Input: part model. Units: mm. Frame: model coordinates. Face numbers are marked on the shaded views. A direction names the side the tool comes from. Round coordinates to 2 decimals unless told otherwise and drop trailing zeros. Order: outer loops, then holes, each group sorted by start corner. A loop starts at its lowest first (then second) coordinate and runs counter-clockwise, first axis right, second up. Notation, with made-up numbers: (87, 27.5) - (129, 27.5) arc R18 cw to (129, 39.5) - close; hole circle Ø7 at (-3, -24.5). An arc over 180 degrees is marked (long way). One line per item, written item: value. Start each with the question number.
from build123d import *

# Parameters (mm, degrees)
F0_R      = 37.5
F0_R_2    = 23.25
F1_DEPTH  = 2.6
F2_R      = 28.25
F2_R_2    = 23.25
F3_DEPTH  = 10
F4_SIZE   = 2
F5_R      = 23.25
F5_R_2    = 4.25
F6_DEPTH  = 2.6
F8_DEPTH  = 2.601
F10_DEPTH = 2.601


with BuildPart() as f1:
    # F0 (on Top) → F1 (new body)
    with BuildSketch(Plane.XY):
        Circle(F0_R)
        Circle(F0_R_2, mode=Mode.SUBTRACT)
    extrude(amount=F1_DEPTH)

    # F2 (on face) → F3 (join)
    with BuildSketch(Plane.XY.offset(2.6)):
        Circle(F2_R)
        Circle(F2_R_2, mode=Mode.SUBTRACT)
    extrude(amount=F3_DEPTH)

    # F4
    f4_edges = [f1.edges().sort_by_distance(p)[0] for p in [
        (-28.25, 0, 12.6),
    ]]
    chamfer(f4_edges, length=F4_SIZE)

    # F5 (on Top) → F6 (join)
    with BuildSketch(Plane.XY):
        Circle(F5_R)
        Circle(F5_R_2, mode=Mode.SUBTRACT)
    extrude(amount=F6_DEPTH)

    # F7 (on face) → F8 (cut, through all)
    with BuildSketch(Plane.XY.offset(2.6)):
        with BuildLine():
            ThreePointArc((-3.877788, 8.121746), (0, 9), (3.877788, 8.121746))
            ThreePointArc((3.877788, 8.121746), (5.806341, 7.897177), (7.468517, 8.900632))
            Line((7.468517, 8.900632), (10.1022, 12.039333))
            ThreePointArc((10.1022, 12.039333), (10.754749, 14.509432), (9.267329, 16.586639))
            ThreePointArc((9.267329, 16.586639), (0, 19), (-9.267329, 16.586639))
            ThreePointArc((-9.267329, 16.586639), (-10.754749, 14.509432), (-10.1022, 12.039333))
            Line((-10.1022, 12.039333), (-7.468517, 8.900632))
            ThreePointArc((-7.468517, 8.900632), (-5.806341, 7.897177), (-3.877788, 8.121746))
        make_face()
        with BuildLine():
            Line((8.900632, -7.468517), (12.039333, -10.1022))
            ThreePointArc((12.039333, -10.1022), (14.509432, -10.754749), (16.586639, -9.267329))
            ThreePointArc((16.586639, -9.267329), (19, 0), (16.586639, 9.267329))
            ThreePointArc((16.586639, 9.267329), (14.509432, 10.754749), (12.039333, 10.1022))
            Line((12.039333, 10.1022), (8.900632, 7.468517))
            ThreePointArc((8.900632, 7.468517), (7.897177, 5.806341), (8.121746, 3.877788))
            ThreePointArc((8.121746, 3.877788), (9, 0), (8.121746, -3.877788))
            ThreePointArc((8.121746, -3.877788), (7.897177, -5.806341), (8.900632, -7.468517))
        make_face()
        with BuildLine():
            Line((-7.468517, -8.900632), (-10.1022, -12.039333))
            ThreePointArc((-10.1022, -12.039333), (-10.754749, -14.509432), (-9.267329, -16.586639))
            ThreePointArc((-9.267329, -16.586639), (0, -19), (9.267329, -16.586639))
            ThreePointArc((9.267329, -16.586639), (10.754749, -14.509432), (10.1022, -12.039333))
            Line((10.1022, -12.039333), (7.468517, -8.900632))
            ThreePointArc((7.468517, -8.900632), (5.806341, -7.897177), (3.877788, -8.121746))
            ThreePointArc((3.877788, -8.121746), (0, -9), (-3.877788, -8.121746))
            ThreePointArc((-3.877788, -8.121746), (-5.806341, -7.897177), (-7.468517, -8.900632))
        make_face()
        with BuildLine():
            Line((-8.900632, 7.468517), (-12.039333, 10.1022))
            ThreePointArc((-12.039333, 10.1022), (-14.509432, 10.754749), (-16.586639, 9.267329))
            ThreePointArc((-16.586639, 9.267329), (-19, 0), (-16.586639, -9.267329))
            ThreePointArc((-16.586639, -9.267329), (-14.509432, -10.754749), (-12.039333, -10.1022))
            Line((-12.039333, -10.1022), (-8.900632, -7.468517))
            ThreePointArc((-8.900632, -7.468517), (-7.897177, -5.806341), (-8.121746, -3.877788))
            ThreePointArc((-8.121746, -3.877788), (-9, 0), (-8.121746, 3.877788))
            ThreePointArc((-8.121746, 3.877788), (-7.897177, 5.806341), (-8.900632, 7.468517))
        make_face()
    extrude(amount=-F8_DEPTH, mode=Mode.SUBTRACT)

    # F9 (on face) → F10 (cut, through all)
    with BuildSketch(Plane.XY.offset(2.6)):
        with BuildLine():
            ThreePointArc((20.688934, 26.962344), (20.884999, 27.716199), (20.480745, 28.38202))
            ThreePointArc((20.480745, 28.38202), (0, 35), (-20.480745, 28.38202))
            ThreePointArc((-20.480745, 28.38202), (-20.884999, 27.716199), (-20.688934, 26.962344))
            Line((-20.688934, 26.962344), (-19.318586, 25.176472))
            ThreePointArc((-19.318586, 25.176472), (-18.671358, 24.795967), (-17.941761, 24.9731))
            ThreePointArc((-17.941761, 24.9731), (0, 30.75), (17.941761, 24.9731))
            ThreePointArc((17.941761, 24.9731), (18.671358, 24.795967), (19.318586, 25.176472))
            Line((19.318586, 25.176472), (20.688934, 26.962344))
        make_face()
        with BuildLine():
            ThreePointArc((26.962344, -20.688934), (27.716199, -20.884999), (28.38202, -20.480745))
            ThreePointArc((28.38202, -20.480745), (35, 0), (28.38202, 20.480745))
            ThreePointArc((28.38202, 20.480745), (27.716199, 20.884999), (26.962344, 20.688934))
            Line((26.962344, 20.688934), (25.176472, 19.318586))
            ThreePointArc((25.176472, 19.318586), (24.795967, 18.671358), (24.9731, 17.941761))
            ThreePointArc((24.9731, 17.941761), (30.75, 0), (24.9731, -17.941761))
            ThreePointArc((24.9731, -17.941761), (24.795967, -18.671358), (25.176472, -19.318586))
            Line((25.176472, -19.318586), (26.962344, -20.688934))
        make_face()
        with BuildLine():
            ThreePointArc((-20.688934, -26.962344), (-20.884999, -27.716199), (-20.480745, -28.38202))
            ThreePointArc((-20.480745, -28.38202), (0, -35), (20.480745, -28.38202))
            ThreePointArc((20.480745, -28.38202), (20.884999, -27.716199), (20.688934, -26.962344))
            Line((20.688934, -26.962344), (19.318586, -25.176472))
            ThreePointArc((19.318586, -25.176472), (18.671358, -24.795967), (17.941761, -24.9731))
            ThreePointArc((17.941761, -24.9731), (0, -30.75), (-17.941761, -24.9731))
            ThreePointArc((-17.941761, -24.9731), (-18.671358, -24.795967), (-19.318586, -25.176472))
            Line((-19.318586, -25.176472), (-20.688934, -26.962344))
        make_face()
        with BuildLine():
            ThreePointArc((-26.962344, 20.688934), (-27.716199, 20.884999), (-28.38202, 20.480745))
            ThreePointArc((-28.38202, 20.480745), (-35, 0), (-28.38202, -20.480745))
            ThreePointArc((-28.38202, -20.480745), (-27.716199, -20.884999), (-26.962344, -20.688934))
            Line((-26.962344, -20.688934), (-25.176472, -19.318586))
            ThreePointArc((-25.176472, -19.318586), (-24.795967, -18.671358), (-24.9731, -17.941761))
            ThreePointArc((-24.9731, -17.941761), (-30.75, 0), (-24.9731, 17.941761))
            ThreePointArc((-24.9731, 17.941761), (-24.795967, 18.671358), (-25.176472, 19.318586))
            Line((-25.176472, 19.318586), (-26.962344, 20.688934))
        make_face()
    extrude(amount=-F10_DEPTH, mode=Mode.SUBTRACT)


solid = f1.part
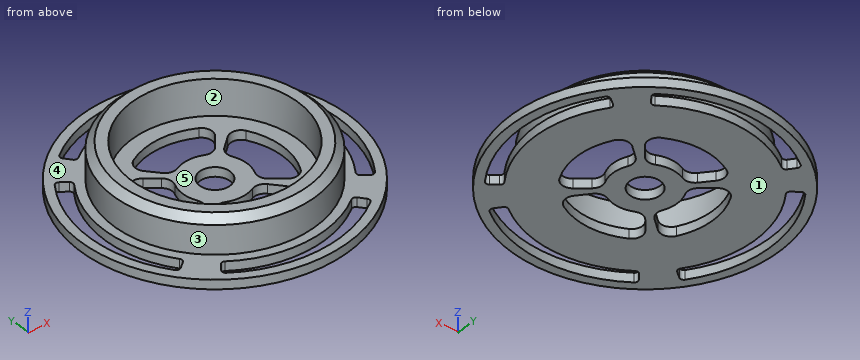
1. Pull-direction query (X, two-part tool) for the marked faces 3, 4 and 5; classes: released by +X, released by -X, zero draft, split by the parting line, or undercut.
2. Set-up query: the marked faces 1 and 2. Return all of +Z, -Z, +X, -X, +Y, -Y with unobstructed straight access to the full face (end or side cutting, diameter ignored); none if empty.
3. Line query: line 1 (Y direction, x = 0, z = 5.75); line 2 (X direction, y = 10.5, z = 2.5); line 3 (Y direction, x = 5.5, z = 2.5). Output: solid intervals per line, ascending. Write a range as from..to.
4. Section A-A (x = 0). State how many separate pieces and enclosed holes the cut face has, then the cut area to 3 significant figures.
5. Section C-C (x = -32). Return the cut outline in (y, z).
6. Pin query (flat end, axial travel): pin 1 (4 mm diameter, centred on y = 17.5, z = 9, fed in from +X); pin 2 (1.5 mm diameter, centred on x = -4, y = 5.5, fed in from +Z); pin 3 (4 mm diameter, centred on x = 14.5, z = 2.5, fed in from +Y). Return the tip coordinate at first contact, or that it passes through.
Solved:
1. face 3: split by the parting line
1. face 4: zero draft
1. face 5: undercut
2. face 1: -Z, +X, -X, +Y, -Y
2. face 2: +Z
3. line 1: y = -28.25..-23.25, 23.25..28.25
3. line 2: x = -36..-33.39, -28.9..-15.28, -12.65..-8.81, 8.81..12.65, 15.28..28.9, 33.39..36
3. line 3: y = -37.09..-34.57, -30.25..-18.19, -7.85..7.85, 18.19..30.25, 34.57..37.09
4. separate pieces: 6
4. enclosed holes: 0
4. area: 195 mm²
5. outline: (-19.55, 0) - (-14.18, 0) - (-14.18, 2.6) - (-19.55, 2.6) - close; (14.18, 0) - (19.55, 0) - (19.55, 2.6) - (14.18, 2.6) - close
6. pin 1: stops at x = 23.62
6. pin 2: stops at z = 2.6
6. pin 3: stops at y = 35.36
